Part model, mm, in its own coordinate system. A direction names the side the tool comes from. Coordinates: 2 decimals unless noted, no trailing zeros. Loops run counter-clockwise (first coordinate to the right, second up) from the corner with the lowest first, then second, coordinate; pieces in that order, holes last. Notation, with made-up numbers: (42, -4.5) - (63, -4.5) arc R10 cw to (63, 10.5) - close; hole circle Ø10 at (-25.5, 61). An arc over 180 degrees is marked (long way). Use a Markdown table: item, result. Add a question column.
1) Band-saw the part on B-B (y = 32). Give the cut face in (x, z) (3 decimals), plus the area to 3 significant figures.
2) Tool access for faces 4 (the face through (30.226, 17, 8)), 5 (the face through (15, 37.465, 8)), 6 (the face through (10.098, 129.804, 3.223)): list every direction of +Z, -Z, +X, -X, +Y, -Y with a clear straight run to the whole face (end or side of a thin tool).
3) Drop flat-ended pins along their axis: P1, Ø2.5, axis at x = 8.52, z = 3.72, coming from the -Y side; P2, Ø8.5, axis at y = 9, z = 5.5, coming from the -X side. Give the stop position or say it passes through.
4) Pull direction Y, two halves, no side cores. Call faces 1 (the face through (15, 34.29, 8)), 2 (the face through (28.62, 7.07, 4.88)), 3 (the face through (20.054, 129.804, 3.646)): +Y half, -Y half, draft (parallel to the pull), parting line (faces both ways), or undercut.
5) Probe probe 1 along Y at (x, z) = (28.5, 8) (3 decimals); probe 2 along Y at (x, z) = (14, 14) (3 decimals); probe 3 along X at (y, z) = (72.5, 5.5). List the from-to ranges inside material, lowest first. Write a range as [from, to].
6) Band-saw the part on A-A (x = -6). Give the cut face in (y, z) (3 decimals).
from build123d import *

# Parameters (mm, degrees)
SKETCH1_W           = 63.5
SKETCH1_H           = 90.7288
BOSS_EXTRUDE1_DEPTH = 16.51
SKETCH2_R           = 3.3782
CUT_EXTRUDE1_DEPTH  = 42.672
SKETCH3_R           = 1.65
CUT_EXTRUDE2_DEPTH  = 42.672


with BuildPart() as part:
    # Sketch1 → Boss-Extrude1 (new body)
    with BuildSketch(Plane.XY):
        Polygon((3.175, 34.29), (27.051, 34.29), (27.051, 0), (30.226, 0), (30.226, 34.29), (50.038, 34.29), (50.038, 131.3688), (-19.812, 131.3688), (-19.812, 34.29), (0, 34.29), (0, 0), (3.175, 0), align=None)
        with Locations((15.113, 82.8294)):
            Rectangle(SKETCH1_W, SKETCH1_H, mode=Mode.SUBTRACT)
    extrude(amount=BOSS_EXTRUDE1_DEPTH)

    # Sketch2 → Cut-Extrude1 (cut)
    with BuildSketch(Plane.ZY):
        with Locations((8.255, 6.9215)):
            Circle(SKETCH2_R)
    extrude(amount=-CUT_EXTRUDE1_DEPTH, mode=Mode.SUBTRACT)

    # Sketch3 → Cut-Extrude2 (cut)
    with BuildSketch(Plane(origin=(0, 131.3688, 0), x_dir=(1, 0, 0), z_dir=(0, 1, 0))):
        with Locations((8.52383023, -3.718168314)):
            Circle(SKETCH3_R)
        with Locations((8.52383023, -12.791831686)):
            Circle(SKETCH3_R)
        with Locations((21.70216977, -12.791831686)):
            Circle(SKETCH3_R)
        with Locations((21.70216977, -3.718168314)):
            Circle(SKETCH3_R)
    extrude(amount=-CUT_EXTRUDE2_DEPTH, mode=Mode.SUBTRACT)


solid = part.part
Answer block:
| question | item | result |
|---|---|---|
| 1 | outline | (0, 0) - (3.175, 0) - (3.175, 16.51) - (0, 16.51) - close; (27.051, 0) - (30.226, 0) - (30.226, 16.51) - (27.051, 16.51) - close |
| 1 | area | 105 mm2 |
| 2 | face 4 | +Z, -Z, +X, -Y |
| 2 | face 5 | +Z, -Z |
| 2 | face 6 | +Y |
| 3 | P1 | y = 34.29 |
| 3 | P2 | x = 0 |
| 4 | face 1 | -Y half |
| 4 | face 2 | undercut |
| 4 | face 3 | draft |
| 5 | probe 1 | [0, 3.553], [10.29, 37.465], [128.194, 131.369] |
| 5 | probe 2 | [34.29, 37.465], [128.194, 131.369] |
| 5 | probe 3 | [-19.81, -16.64], [46.86, 50.04] |
| 6 | outline | (34.29, 0) - (37.465, 0) - (37.465, 16.51) - (34.29, 16.51) - close; (128.194, 0) - (131.369, 0) - (131.369, 16.51) - (128.194, 16.51) - close |
